from build123d import *

# Parameters (mm, degrees)
F0_W     = 254
F0_H     = 38.1
F0_R     = 3.175
F1_DEPTH = 3.175


with BuildPart() as f1:
    # F0 (on Right) → F1 (new body)
    with BuildSketch(Plane.YZ):
        Rectangle(F0_W, F0_H)
        with BuildLine():
            ThreePointArc((127, -19.05), (146.05, 0), (127, 19.05))
            Line((127, 19.05), (127, -19.05))
        make_face()
        with Locations((133.35, 0)):
            Circle(F0_R, mode=Mode.SUBTRACT)
        with BuildLine():
            Line((-127, -19.05), (-127, 19.05))
            ThreePointArc((-127, 19.05), (-146.05, 0), (-127, -19.05))
        make_face()
        with Locations((-133.35, 0)):
            Circle(F0_R, mode=Mode.SUBTRACT)
    extrude(amount=F1_DEPTH)


solid = f1.part
The model under review builds one solid part; all positions refer to its coordinate system, in mm. Round coordinates to 2 decimals unless told otherwise and drop trailing zeros. Loops run counter-clockwise (first coordinate to the right, second up) from the corner with the lowest first, then second, coordinate; pieces in that order, holes last. Notation, with made-up numbers: M 43.5,-26 L 64.5,-26 A17 ccw 64.5,-22 Z; hole C 83,-29.75 d7. An arc over 180 degrees is marked long. Answer as CSV lines item,"result". Start each with the question number.
Item 1: Consider section A-A (z = 0). Write out the cut boundary in (x, y) (3 decimals), then the cut area to 3 significant figures.
Item 2: Wall thickness on line 1 (Y direction, x = 2.7, z = 2); line 2 (Y direction, x = 1.2, z = 16); line 3 (Y direction, x = 1.8, z = 15.5): over which ranges is each line inside the solid? List them lowest first. Write a range as [from, to].
Item 3: Consider section C-C (y = 133.35). Write out the cut boundary in (x, z) (3 decimals).
Item 4: Mouldability with a two-part tool opening along Y and no side actions: class faces 1 (the face through (1.57, -130.42, -1.22)), 2 (the face through (0, -2, 0)), 3 (the face through (1.565, 146.045, -0.419)) as released by +Y, released by -Y, zero draft, split by the parting line, or undercut.
Item 5: Consider section B-B (x = 2.15). Write out the cut boundary in (y, z) (3 decimals).
Item 6: Consider section D-D (z = 12.5). Write out the cut boundary in (x, y) (3 decimals).
Answer:
1,outline,"M 0,-146.05 L 3.175,-146.05 L 3.175,-136.525 L 0,-136.525 Z; M 0,-130.175 L 3.175,-130.175 L 3.175,130.175 L 0,130.175 Z; M 0,136.525 L 3.175,136.525 L 3.175,146.05 L 0,146.05 Z"
1,area,"887 mm^2"
2,line 1,"y = [-145.94, -135.82], [-130.88, 130.88], [135.82, 145.94]"
2,line 2,"y = [-137.34, 137.34]"
2,line 3,"y = [-138.07, 138.07]"
3,outline,"M 0,-17.961 L 3.175,-17.961 L 3.175,-3.175 L 0,-3.175 Z; M 0,3.175 L 3.175,3.175 L 3.175,17.961 L 0,17.961 Z"
4,face 1,"undercut"
4,face 2,"zero draft"
4,face 3,"released by +Y"
5,outline,"M -127,-19.05 L 127,-19.05 A19.05 ccw 127,19.05 L -127,19.05 A19.05 ccw Z; hole C -133.35,0 d6.35; hole C 133.35,0 d6.35"
6,outline,"M 0,-141.375 L 3.175,-141.375 L 3.175,141.375 L 0,141.375 Z"
